The drawing under review shows one solid part. Ordinate dimensions are in mm from its lowest x, y, z. A direction names the side the tool comes from. Coordinates: 2 decimals unless noted, no trailing zeros. Order: outer loops, then holes, each group sorted by start corner. A loop starts at its lowest first (then second) coordinate and runs counter-clockwise, first axis right, second up. Notation, with made-up numbers: (-11, -22) - (30, -22) arc R16 cw to (30, 6) - close; hole circle Ø7 at (9.5, 13). An arc over 180 degrees is marked (long way). Write each question's results on one line, items separated by ' | '. Start each with the question number.
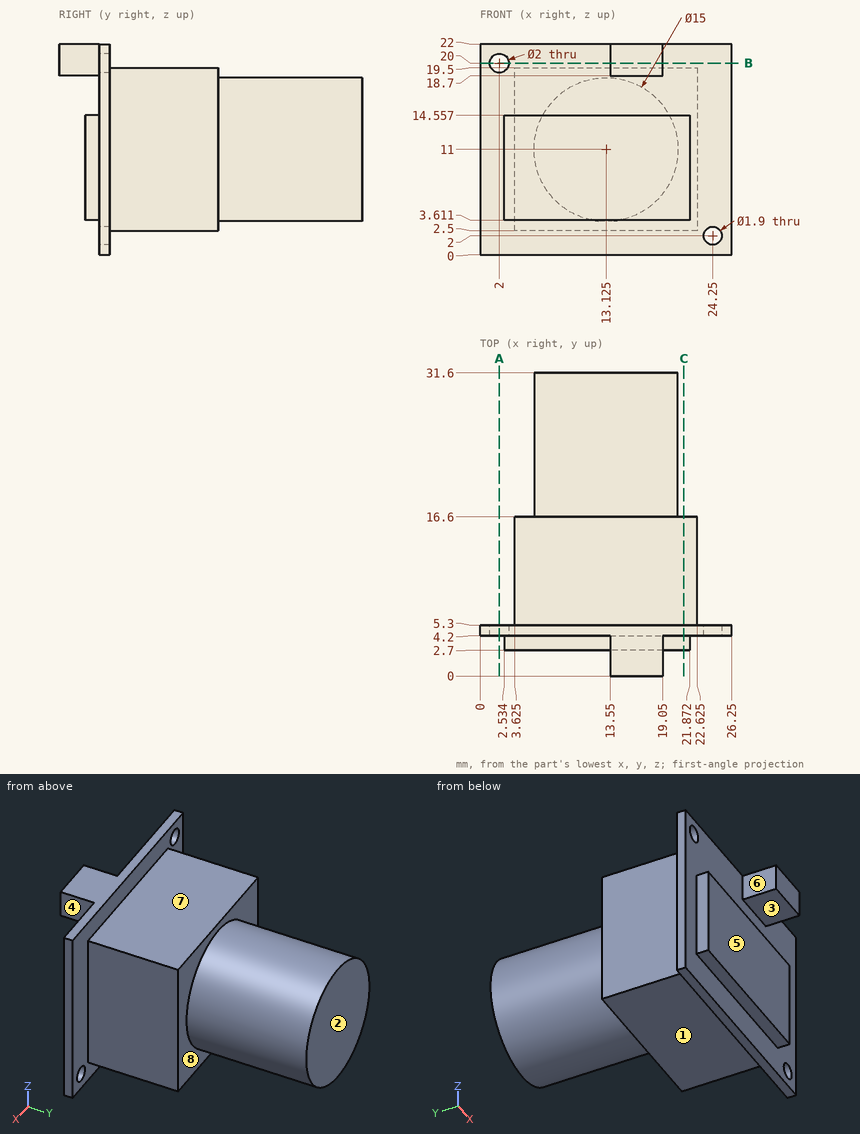
(1) Take a section at B-B (z = 20). State the section outline as (x, y) points.
(2) Clearance check with flat-ended pins moving along their axes: pin 1 (1 mm diameter, centred on y = 2, z = 21, fed in from -X); pin 2 (5 mm diameter, centred on x = 3.5, z = 12, fed in from -Y); pin 3 (5.5 mm diameter, centred on x = 8.5, y = 10.5, fed in from +Z); pin 4 (1.5 mm diameter, centred on x = 24.25, z = 2, fed in from +Y). State where each tip first meets the part, or that it passes through.
(3) Take a section at C-C (x = 21.25). State the section outline as (y, z) points, plus the area to 3 significant figures.
(4) Mouldability with a two-part tool opening along Z and no side actions: class the marked faces 1, 2 and 3 as +Z half, -Z half, draft (parallel to the pull), parting line (faces both ways), or undercut.
(5) To check wall thickness, follow line 1 along Z through (x, y) = (2, 5.15); line 2 along Y through (x, z) = (12.25, 17.25); line 3 along Y through (x, z) = (15.75, 8). State the ranges of each line that lie inside material, in increasing order. Write a range as [from, to].
(6) Take a section at A-A (x = 2). State the section outline as (y, z) points, plus the area to 3 significant figures.
(7) Tool access review of the marked faces 4, 5, 6, 7 and 8: name each direction out of +Z, -Z, +X, -X, +Y, -Y from which nothing blocks a thin tool from reaching the whole face with its end or side.
Worked out:
1) outline: (0, 4.2) - (1, 4.2) - (1, 5.3) - (0, 5.3) - close; (3, 4.2) - (13.55, 4.2) - (13.55, 0) - (19.05, 0) - (19.05, 4.2) - (26.25, 4.2) - (26.25, 5.3) - (3, 5.3) - close
2) pin 1: x = 13.55 | pin 2: y = 2.7 | pin 3: z = 19.5 | pin 4: through
3) outline: (2.7, 3.61) - (4.2, 3.61) - (4.2, 0) - (5.3, 0) - (5.3, 2.5) - (16.6, 2.5) - (16.6, 19.5) - (5.3, 19.5) - (5.3, 22) - (4.2, 22) - (4.2, 14.56) - (2.7, 14.56) - close | area: 233 mm^2
4) face 1: -Z half | face 2: draft | face 3: undercut
5) line 1: [0, 19], [21, 22] | line 2: [4.2, 31.6] | line 3: [2.7, 31.6]
6) outline: (4.2, 0) - (5.3, 0) - (5.3, 19) - (4.2, 19) - close; (4.2, 21) - (5.3, 21) - (5.3, 22) - (4.2, 22) - close | area: 22.0 mm^2
7) face 4: +Z, +X, -Y | face 5: -Z, +X, -X, -Y | face 6: +Z, -X, -Y | face 7: +Z, +X, -X, +Y | face 8: +Y
